Check sheet for the drawn part. Datum: minimum x, y, z corner. Units: mm. A direction names the side the tool comes from. Give positions to 0.01 mm unless a question says otherwise; leave off trailing zeros. Loops run counter-clockwise (first coordinate to the right, second up) from the corner with the lowest first, then second, coordinate; pieces in that order, holes last. Notation, with made-up numbers: (6, -35) - (24, -35) arc R21 cw to (24, -18) - close; hole circle Ø5 at (-13.5, 18.25). An arc over 180 degrees is marked (long way). Answer in a Markdown table with one row per item.
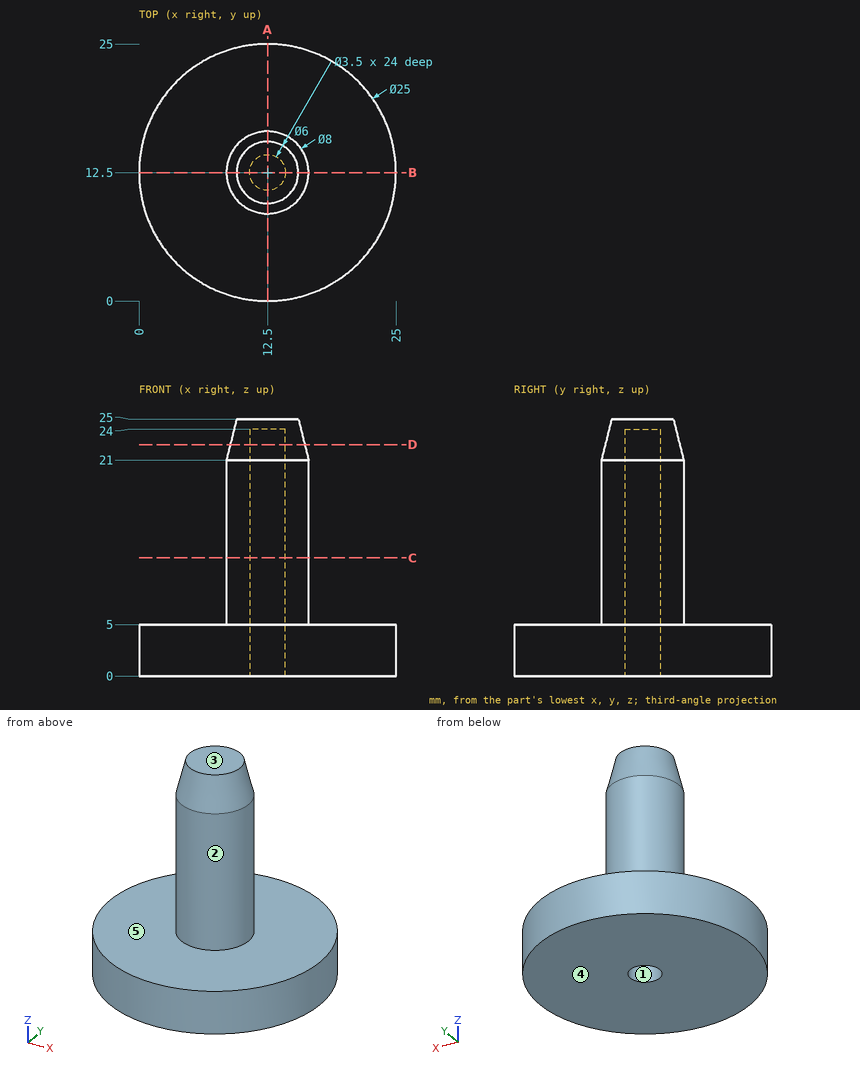
Q1. Tool access check on the marked faces 4 and 5. Record the directions out of +Z, -Z, +X, -X, +Y, -Y that give a thin tool (end or side, any length) a straight path to the whole face; none if there is none.
Completed:
| item | result |
|---|---|
| face 4 | -Z, +X, -X, +Y, -Y |
| face 5 | +Z |
Q2. Draft check along X on the marked faces 1, 2 and 3. Enter one of: +X half, -X half, draft (parallel to the pull), parting line (faces both ways), or undercut.
Completed:
| item | result |
|---|---|
| face 1 | undercut |
| face 2 | parting line |
| face 3 | draft |
Q3. Sectioned sample at C-C (z = 11.5). Record the cut outline in (x, y), and give its area (3 significant figures).
Completed:
| item | result |
|---|---|
| outline | circle Ø8 at (12.5, 12.5); hole circle Ø3.5 at (12.5, 12.5) |
| area | 40.6 mm^2 |
Q4. Sectioned sample at D-D (z = 22.5). Record the cut outline in (x, y) (3 decimals).
Completed:
| item | result |
|---|---|
| outline | circle Ø7.25 at (12.5, 12.5); hole circle Ø3.5 at (12.5, 12.5) |
Q5. Go/stop test with flat-tipped pins: P1, Ø6, axis at x = 16, y = 13.5, coming from the -Z side; P2, Ø2, axis at x = 16, z = 22, coming from the +Y side; P3, Ø8, axis at y = 8.5, z = 20, coming from the -X side; P4, Ø1.8, axis at x = 12.5, y = 13, coming from the -Z side. Record where each tip stops, or that it passes through.
Completed:
| item | result |
|---|---|
| P1 | z = 0 |
| P2 | y = 15.36 |
| P3 | x = 8.5 |
| P4 | z = 24 |
Q6. Sectioned sample at A-A (x = 12.5). Record the cut outline in (y, z), and give its area (3 significant figures).
Completed:
| item | result |
|---|---|
| outline | (0, 0) - (10.75, 0) - (10.75, 24) - (14.25, 24) - (14.25, 0) - (25, 0) - (25, 5) - (16.5, 5) - (16.5, 21) - (15.5, 25) - (9.5, 25) - (8.5, 21) - (8.5, 5) - (0, 5) - close |
| area | 197 mm^2 |
Q7. Thickness scan on line 1 (Y direction, x = 12.5, z = 14.5); line 2 (Z direction, x = 3, y = 8.5); line 3 (X direction, y = 13.25, z = 15.5). Record the ranges inside material, lowest first.
Completed:
| item | result |
|---|---|
| line 1 | 8.5 to 10.75, 14.25 to 16.5 |
| line 2 | 0 to 5 |
| line 3 | 8.57 to 10.92, 14.08 to 16.43 |
